Geometry: final body of the model. Coordinates: model frame, mm. A direction names the side the tool comes from. Round coordinates to 2 decimals unless told otherwise and drop trailing zeros. Loops run counter-clockwise (first coordinate to the right, second up) from the corner with the lowest first, then second, coordinate; pieces in that order, holes last. Notation, with made-up numbers: M 16,31 L 61,31 A25 cw 61,46 Z; hole C -1.5,2.25 d6. An arc over 180 degrees is marked long. Answer as a JSON object with one key per item and string values.
from build123d import *

# Parameters (mm, degrees)
F0_R     = 11.176
F1_DEPTH = 3.556


with BuildPart() as f1:
    # F0 (on Front) → F1 (new body, symmetric)
    with BuildSketch(Plane.XZ):
        with BuildLine():
            ThreePointArc((6.7002799246, -9.8976827694), (10.5579766794, -5.6024105266), (11.9523167324, 0))
            ThreePointArc((11.9523167324, 0), (11.9304871649, 0.7220465922), (11.8650782007, 1.4414557099))
            ThreePointArc((11.8650782007, 1.4414557099), (11.3793199415, 3.6563578792), (10.4839962384, 5.7396601071))
            Line((10.4839962384, 5.7396601071), (9.8030486125, 5.3668625751))
            ThreePointArc((9.8030486125, 5.3668625751), (10.8273230139, 2.7698469909), (11.176, 0))
            ThreePointArc((11.176, 0), (7.9026253865, -7.9026253865), (0, -11.176))
            Line((0, -11.176), (0, -11.9523167324))
            ThreePointArc((0, -11.9523167324), (3.5041144313, -11.42711938), (6.7002799246, -9.8976827694))
        make_face()
        with BuildLine():
            ThreePointArc((10.4839962384, 5.7396601071), (11.3793199415, 3.6563578792), (11.8650782007, 1.4414557099))
            ThreePointArc((11.8650782007, 1.4414557099), (15.1468517315, 2.0483664496), (18.4490286697, 1.5646251732))
            ThreePointArc((18.4490286697, 1.5646251732), (15.1517773463, 3.8060939797), (12.7119618322, 6.9594016014))
            Line((12.7119618322, 6.9594016014), (10.4839962384, 5.7396601071))
        make_face()
        with BuildLine():
            ThreePointArc((9.1344120356, -18.3689094107), (6.9562324961, -14.4094635558), (6.7002799246, -9.8976827694))
            ThreePointArc((6.7002799246, -9.8976827694), (3.5041144313, -11.42711938), (0, -11.9523167324))
            Line((0, -11.9523167324), (0, -14.4923167324))
            ThreePointArc((0, -14.4923167324), (4.9614880336, -15.5015666926), (9.1344120356, -18.3689094107))
        make_face()
        with BuildLine():
            Line((9.8030486125, 5.3668625751), (10.4839962384, 5.7396601071))
            ThreePointArc((10.4839962384, 5.7396601071), (9.2113316577, 7.6163800039), (7.6071320504, 9.2189705087))
            ThreePointArc((7.6071320504, 9.2189705087), (4.0416469295, 11.2482427681), (0, 11.9523167324))
            Line((0, 11.9523167324), (0, 11.176))
            ThreePointArc((0, 11.176), (5.6974959351, 9.6146511153), (9.8030486125, 5.3668625751))
        make_face()
        with BuildLine():
            ThreePointArc((7.6071320504, 9.2189705087), (9.2113316577, 7.6163800039), (10.4839962384, 5.7396601071))
            Line((10.4839962384, 5.7396601071), (12.7119618322, 6.9594016014))
            ThreePointArc((12.7119618322, 6.9594016014), (11.3700398508, 10.7137716013), (11.2582654612, 14.6991894196))
            ThreePointArc((11.2582654612, 14.6991894196), (9.8866064691, 11.6566691217), (7.6071320504, 9.2189705087))
        make_face()
        with BuildLine():
            ThreePointArc((19.8117182154, 1.0178507045), (19.1402143158, 1.3157636909), (18.4490286697, 1.5646251732))
            ThreePointArc((18.4490286697, 1.5646251732), (19.1224650067, 1.2715282716), (19.8117182154, 1.0178507045))
        make_face()
        with BuildLine():
            ThreePointArc((12.7119618322, 6.9594016014), (15.1517773463, 3.8060939797), (18.4490286697, 1.5646251732))
            ThreePointArc((18.4490286697, 1.5646251732), (19.1402143158, 1.3157636909), (19.8117182154, 1.0178507045))
            ThreePointArc((19.8117182154, 1.0178507045), (31.2673508338, 2.7479463892), (36.551789801, 13.0581090731))
            ThreePointArc((36.551789801, 13.0581090731), (25.4052864941, 25.6627371131), (11.5318452302, 16.1417701721))
            ThreePointArc((11.5318452302, 16.1417701721), (11.4210189836, 15.415555894), (11.2582654612, 14.6991894196))
            ThreePointArc((11.2582654612, 14.6991894196), (11.3700398508, 10.7137716013), (12.7119618322, 6.9594016014))
        make_face()
        with BuildLine():
            ThreePointArc((35.027789801, 13.0581090731), (26.6216367919, 2.2307860593), (14.0487411884, 7.691246498))
            ThreePointArc((14.0487411884, 7.691246498), (21.0819428101, 23.885432087), (35.027789801, 13.0581090731))
        make_face(mode=Mode.SUBTRACT)
        with BuildLine():
            Line((0, -14.4923167324), (0, -11.9523167324))
            ThreePointArc((0, -11.9523167324), (-3.5041144313, -11.42711938), (-6.7002799246, -9.8976827694))
            ThreePointArc((-6.7002799246, -9.8976827694), (-6.9562324961, -14.4094635558), (-9.1344120356, -18.3689094107))
            ThreePointArc((-9.1344120356, -18.3689094107), (-4.9614880336, -15.5015666926), (0, -14.4923167324))
        make_face()
        with BuildLine():
            ThreePointArc((-6.7002799246, -9.8976827694), (-3.5041144313, -11.42711938), (0, -11.9523167324))
            Line((0, -11.9523167324), (0, -11.176))
            ThreePointArc((0, -11.176), (-11.176, 0), (0, 11.176))
            Line((0, 11.176), (0, 11.9523167324))
            ThreePointArc((0, 11.9523167324), (-4.0416469295, 11.2482427681), (-7.6071320504, 9.2189705087))
            ThreePointArc((-7.6071320504, 9.2189705087), (-10.4839962384, 5.7396601071), (-11.8650782007, 1.4414557099))
            ThreePointArc((-11.8650782007, 1.4414557099), (-10.8771386837, -4.9543646745), (-6.7002799246, -9.8976827694))
        make_face()
        with BuildLine():
            ThreePointArc((9.4583258088, -18.7170543238), (9.2943419701, -18.544867742), (9.1344120356, -18.3689094107))
            ThreePointArc((9.1344120356, -18.3689094107), (4.9614880336, -15.5015666926), (0, -14.4923167324))
            ThreePointArc((0, -14.4923167324), (-4.9614880336, -15.5015666926), (-9.1344120356, -18.3689094107))
            ThreePointArc((-9.1344120356, -18.3689094107), (-9.2943419701, -18.544867742), (-9.4583258088, -18.7170543238))
            ThreePointArc((-9.4583258088, -18.7170543238), (-4.5370288862, -39.0542461238), (12.7, -27.1923167324))
            ThreePointArc((12.7, -27.1923167324), (11.8619293914, -22.6552878462), (9.4583258088, -18.7170543238))
        make_face()
        with BuildLine():
            ThreePointArc((11.176, -27.1923167324), (-7.9026253865, -35.094942119), (0, -16.0163167324))
            ThreePointArc((0, -16.0163167324), (7.9026253865, -19.2896913459), (11.176, -27.1923167324))
        make_face(mode=Mode.SUBTRACT)
        with BuildLine():
            ThreePointArc((9.4583258088, -18.7170543238), (9.2979985135, -18.5414656967), (9.1344120356, -18.3689094107))
            ThreePointArc((9.1344120356, -18.3689094107), (9.2943419701, -18.544867742), (9.4583258088, -18.7170543238))
        make_face()
        with BuildLine():
            ThreePointArc((11.5318452302, 16.1417701721), (11.3741901482, 15.4244367985), (11.2582654612, 14.6991894196))
            ThreePointArc((11.2582654612, 14.6991894196), (11.4210189836, 15.415555894), (11.5318452302, 16.1417701721))
        make_face()
        with BuildLine():
            ThreePointArc((-18.4490286697, 1.5646251732), (-15.1468517315, 2.0483664496), (-11.8650782007, 1.4414557099))
            ThreePointArc((-11.8650782007, 1.4414557099), (-10.4839962384, 5.7396601071), (-7.6071320504, 9.2189705087))
            ThreePointArc((-7.6071320504, 9.2189705087), (-9.8866064691, 11.6566691217), (-11.2582654612, 14.6991894196))
            ThreePointArc((-11.2582654612, 14.6991894196), (-11.178436671, 13.8803745062), (-11.151789801, 13.0581090731))
            ThreePointArc((-11.151789801, 13.0581090731), (-13.1301978864, 6.2509461681), (-18.4490286697, 1.5646251732))
        make_face()
        with BuildLine():
            ThreePointArc((-9.4583258088, -18.7170543238), (-9.2943419701, -18.544867742), (-9.1344120356, -18.3689094107))
            ThreePointArc((-9.1344120356, -18.3689094107), (-9.2979985135, -18.5414656967), (-9.4583258088, -18.7170543238))
        make_face()
        with BuildLine():
            ThreePointArc((-19.8117182154, 1.0178507045), (-19.1224650067, 1.2715282716), (-18.4490286697, 1.5646251732))
            ThreePointArc((-18.4490286697, 1.5646251732), (-19.1402143158, 1.3157636909), (-19.8117182154, 1.0178507045))
        make_face()
        with BuildLine():
            ThreePointArc((-19.8117182154, 1.0178507045), (-19.1402143158, 1.3157636909), (-18.4490286697, 1.5646251732))
            ThreePointArc((-18.4490286697, 1.5646251732), (-13.1301978864, 6.2509461681), (-11.151789801, 13.0581090731))
            ThreePointArc((-11.151789801, 13.0581090731), (-11.178436671, 13.8803745062), (-11.2582654612, 14.6991894196))
            ThreePointArc((-11.2582654612, 14.6991894196), (-11.4210189836, 15.415555894), (-11.5318452302, 16.1417701721))
            ThreePointArc((-11.5318452302, 16.1417701721), (-34.9916177698, 19.1568165449), (-19.8117182154, 1.0178507045))
        make_face()
        with Locations((-23.851789801, 13.0581090731)):
            Circle(F0_R, mode=Mode.SUBTRACT)
        with BuildLine():
            ThreePointArc((-11.5318452302, 16.1417701721), (-11.4210189836, 15.415555894), (-11.2582654612, 14.6991894196))
            ThreePointArc((-11.2582654612, 14.6991894196), (-11.3741901482, 15.4244367985), (-11.5318452302, 16.1417701721))
        make_face()
    extrude(amount=F1_DEPTH, both=True)


solid = f1.part
1) Section query C-C (y = -1). Return the cut outline in (x, z), and give its area (3 significant figures).
Results:
{"outline": "M -18.45,1.56 A10.21 cw -11.87,1.44 A11.95 ccw -6.7,-9.9 A10.21 cw -9.13,-18.37 A12.7 ccw long 9.13,-18.37 A10.21 cw 6.7,-9.9 A11.95 ccw 11.87,1.44 A10.21 cw 18.45,1.56 A12.7 ccw long 11.26,14.7 A10.21 cw 7.61,9.22 A11.95 ccw -7.61,9.22 A10.21 cw -11.26,14.7 A12.7 ccw long Z; hole C -23.85,13.06 d22.35; hole C 0,-27.19 d22.35; hole C 0,0 d22.35; hole C 23.85,13.06 d22.35", "area": "524 mm2"}
2) Section query B-B (z = 4.5). Return the cut outline in (x, y), and give its area (3 significant figures).
Results:
{"outline": "M -33.24,-3.56 L -31.04,-3.56 L -31.04,3.56 L -33.24,3.56 Z; M -16.66,-3.56 L -10.23,-3.56 L -10.23,3.56 L -16.66,3.56 Z; M 10.23,-3.56 L 16.66,-3.56 L 16.66,3.56 L 10.23,3.56 Z; M 31.04,-3.56 L 33.24,-3.56 L 33.24,3.56 L 31.04,3.56 Z", "area": "123 mm2"}
3) Section query A-A (x = -29.5). Return the cut outline in (y, z), and give its area (3 significant figures).
Results:
{"outline": "M -3.56,1.68 L 3.56,1.68 L 3.56,3.41 L -3.56,3.41 Z; M -3.56,22.7 L 3.56,22.7 L 3.56,24.43 L -3.56,24.43 Z", "area": "24.6 mm2"}
4) Ray query, line 1 (Z direction, x = 2.5, y = 3); line 2 (Z direction, x = -5, y = -1); line 3 (X direction, y = -0.25, z = 12.5). Return the intervals inside material, ascending.
Results:
{"line 1": "-39.64 to -38.09, -16.3 to -10.89, 10.89 to 11.69", "line 2": "-38.87 to -37.19, -17.2 to -10, 10 to 10.86", "line 3": "-36.54 to -35.01, -12.69 to -10.39, 10.39 to 12.69, 35.01 to 36.54"}
5) Section query D-D (z = -34). Return the cut outline in (x, y).
Results:
{"outline": "M -10.72,-3.56 L -8.86,-3.56 L -8.86,3.56 L -10.72,3.56 Z; M 8.86,-3.56 L 10.72,-3.56 L 10.72,3.56 L 8.86,3.56 Z"}
6) Reachability of faces 5 (the cylindrical face through (9.913, 0.05, 11.696)), 6 (the cylindrical face through (-6.94, -0.05, -14.35)) from +Z, -Z, +X, -X, +Y, -Y: full face, straight path, thin tool, end or side. Return the list, or none.
Results:
{"face 5": "+Z, +Y, -Y", "face 6": "-X, +Y, -Y"}
7) Pull-direction query (X, two-part tool) for faces 1 (the cylindrical face through (6.974, -0.05, -14.471)), 2 (the cylindrical face through (-9.86, 0.05, 11.62)), 3 (the flat face through (11, 3.556, -4)), 4 (the cylindrical face through (-15.19, 0.05, 2.05)); classes: +X half, -X half, draft (parallel to the pull), parting line (faces both ways), or undercut.
Results:
{"face 1": "+X half", "face 2": "undercut", "face 3": "draft", "face 4": "undercut"}
8) Pin query (flat end, axial travel): P1, Ø4, axis at x = -16.5, y = -3, coming from the -Z side; P2, Ø3, axis at y = 1.5, z = -9.5, coming from the +X side; P3, Ø13.5, axis at x = 23.85, z = 13.06, coming from the +Y side; P4, Ø3, axis at x = -27.5, y = 0.5, coming from the +Z side. Return the tip coordinate at first contact, or that it passes through.
Results:
{"P1": "z = 1.54", "P2": "x = 8.88", "P3": "through", "P4": "z = 25.58"}
